Can you work these out from the drawing? Everything is in mm from the part's minimum corner. A direction names the side the tool comes from. Coordinates: 2 decimals unless noted, no trailing zeros. Loops run counter-clockwise (first coordinate to the right, second up) from the corner with the lowest first, then second, coordinate; pieces in that order, holes last. Notation, with made-up numbers: (55.25, 1.25) - (112.25, 1.25) arc R8 ccw to (112.25, 6.25) - close; hole circle Ø7 at (76, 0). An arc over 180 degrees is marked (long way). One line per question, with ' | ' between items. Start each with the question number.
1. We'd pull the mould along Y, two halves only. Please class the marked faces 1, 2 and 3: pulls with the +Y half, pulls with the -Y half, needs draft (parallel to the pull), parting line crosses it, or undercut.
2. I want a section at A-A, the plane x = 7.5. Write out the boundary of the cut face in (y, z), then the cut area to 3 significant figures.
3. I want a section at D-D, the plane x = 14.25. Write out the boundary of the cut face in (y, z).
4. I'm going to push flat-ended pins straight in: P1, Ø2, axis at x = 7.5, z = 28, coming from the -Y side; P2, Ø8, axis at x = 8, z = 27.5, coming from the +Y side; P3, Ø1, axis at x = 7, z = 0.5, coming from the +Y side; P4, Ø7, axis at x = 6.5, y = 7, coming from the +Z side. Where does each tip first touch, or does it pass through?
5. I want a section at C-C, the plane y = 6.75. Write out the boundary of the cut face in (x, z), then the cut area to 3 significant figures.
6. Which directions (+Z, -Z, +X, -X, +Y, -Y) give clear straight access to the entire face, cutting with the end or side of a thin tool? Please do the marked faces 4 and 5.
7. Please list where these lines run through material, in increasing order: L1, parallel to Y at x = 2.5, z = 28; L2, parallel to Z at x = 7.5, y = 1.75; L3, parallel to Z at x = 12.25, y = 13.75. Write a range as [from, to].
8. I want a section at B-B, the plane z = 27.8. Write out the boundary of the cut face in (x, y).
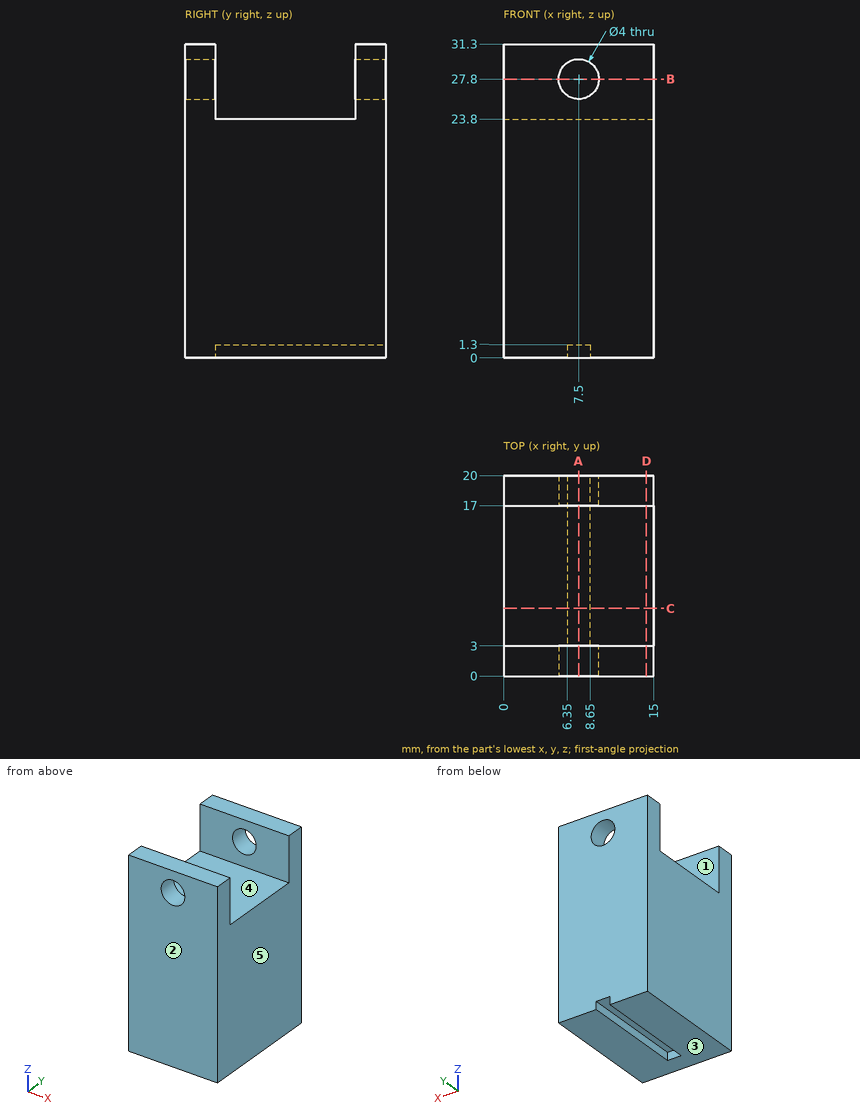
Results are:
1) face 1: undercut | face 2: pulls with the -Y half | face 3: needs draft
2) outline: (0, 0) - (3, 0) - (3, 1.3) - (20, 1.3) - (20, 25.8) - (17, 25.8) - (17, 23.8) - (3, 23.8) - (3, 25.8) - (0, 25.8) - close; (0, 29.8) - (3, 29.8) - (3, 31.3) - (0, 31.3) - close; (17, 29.8) - (20, 29.8) - (20, 31.3) - (17, 31.3) - close | area: 475 mm2
3) outline: (0, 0) - (20, 0) - (20, 31.3) - (17, 31.3) - (17, 23.8) - (3, 23.8) - (3, 31.3) - (0, 31.3) - close
4) P1: passes through | P2: stops at y = 20 | P3: stops at y = 3 | P4: stops at z = 23.8
5) outline: (0, 0) - (6.35, 0) - (6.35, 1.3) - (8.65, 1.3) - (8.65, 0) - (15, 0) - (15, 23.8) - (0, 23.8) - close | area: 354 mm2
6) face 4: +Z, +X, -X | face 5: +Z, -Z, +X, +Y, -Y
7) L1: y = [0, 3], [17, 20] | L2: z = [0, 25.8], [29.8, 31.3] | L3: z = [0, 23.8]
8) outline: (0, 0) - (5.5, 0) - (5.5, 3) - (0, 3) - close; (0, 17) - (5.5, 17) - (5.5, 20) - (0, 20) - close; (9.5, 0) - (15, 0) - (15, 3) - (9.5, 3) - close; (9.5, 17) - (15, 17) - (15, 20) - (9.5, 20) - close
